For this review, use the dimensioned drawing (mm, ordinates from the lowest corner) and the shaded views. A direction names the side the tool comes from. Give positions to 0.01 mm unless a question says otherwise; leave off trailing zeros. Order: outer loops, then holes, each group sorted by start corner. A loop starts at its lowest first (then second) coordinate and runs counter-clockwise, first axis right, second up. Notation, with made-up numbers: (67, 24.5) - (93, 24.5) arc R26 cw to (93, 61.5) - close; hole circle Ø10 at (82, 62). An arc over 180 degrees is marked (long way). Use a Markdown table: item, result. Add a question column.
1) Clearance check with flat-ended pins moving along their axes: P1, Ø16, axis at y = 9.5, z = 26.5, coming from the +X side; P2, Ø1, axis at y = 16.5, z = 10.5, coming from the -X side; P3, Ø6, axis at x = 12, y = 30.5, coming from the +Z side. State where each tip first meets the part, or that it passes through.
2) We need section C-C on x = 32.5. Write out the cut boundary in (y, z), then the cut area to 3 significant figures.
3) We need section D-D on z = 26.5. Write out the cut boundary in (x, y).
4) We need section B-B on z = 8. Write out the cut boundary in (x, y).
5) Mouldability with a two-part tool opening along X and no side actions: class the marked faces 5, 6, 7 and 8 as released by +X, released by -X, zero draft, split by the parting line, or undercut.
6) Wall thickness on L1, parallel to Z at x = 11, y = 40.25; L2, parallel to Z at x = 14, y = 39.5; L3, parallel to Y at x = 31.5, z = 36.5: over which ranges is each line inside the solid? List them lowest first.
7) Machinability: for the marked faces 1, 2, 3 and 4, which of the approach directions +Z, -Z, +X, -X, +Y, -Y give a long, thin tool a straight path to every point of the face, cutting with its end or side? Answer none if there is none.
8) We need section A-A on z = 3. Write out the cut boundary in (x, y), then the cut area to 3 significant figures.
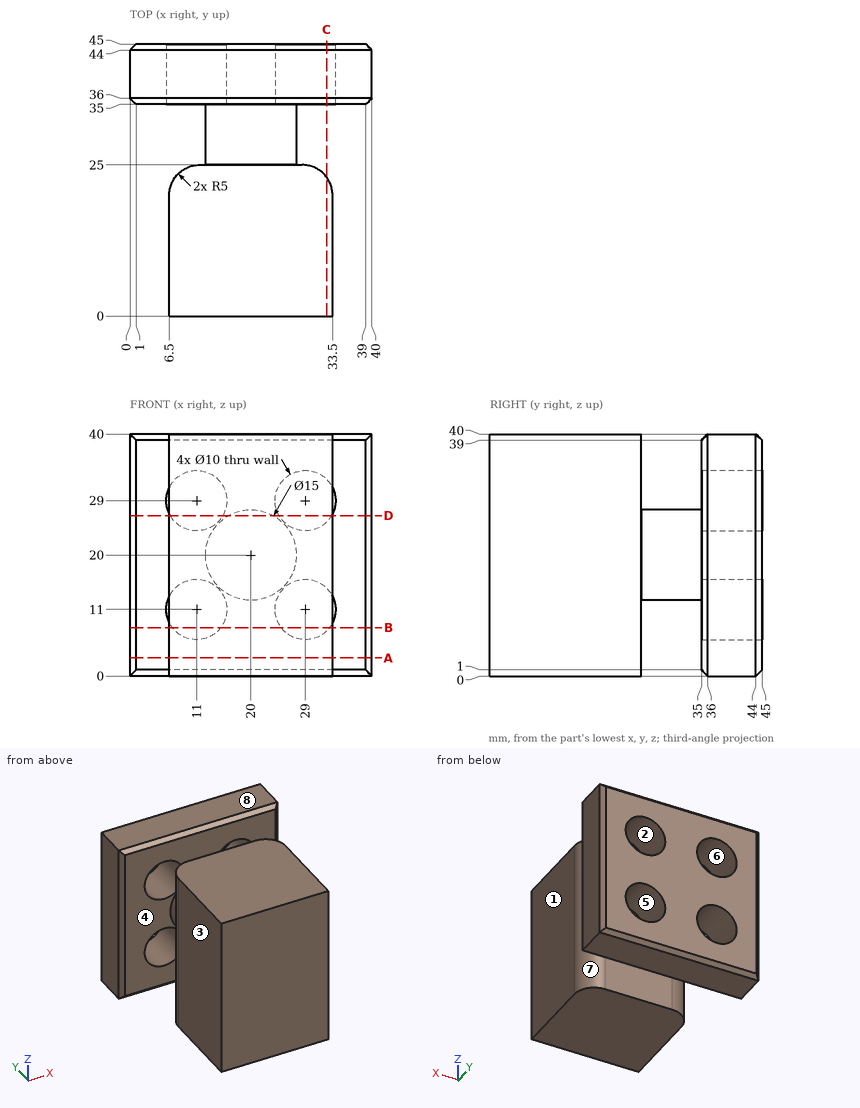
Checked values:
| question | item | result |
|---|---|---|
| 1 | P1 | x = 33.5 |
| 1 | P2 | x = 6.5 |
| 1 | P3 | z = 25.59 |
| 2 | outline | (0, 0) - (23, 0) - (23, 40) - (0, 40) - close; (35, 1) - (36, 0) - (44, 0) - (45, 1) - (45, 7.43) - (35, 7.43) - close; (35, 14.57) - (45, 14.57) - (45, 25.43) - (35, 25.43) - close; (35, 32.57) - (45, 32.57) - (45, 39) - (44, 40) - (36, 40) - (35, 39) - close |
| 2 | area | 1,180 mm² |
| 3 | outline | (0, 36) - (1, 35) - (6.67, 35) - (6.67, 45) - (1, 45) - (0, 44) - close; (6.5, 0) - (33.5, 0) - (33.5, 20) arc R5 ccw to (28.5, 25) - (23.74, 25) - (23.74, 35) - (24.67, 35) - (24.67, 45) - (15.33, 45) - (15.33, 35) - (16.26, 35) - (16.26, 25) - (11.5, 25) arc R5 ccw to (6.5, 20) - close; (33.33, 35) - (39, 35) - (40, 36) - (40, 44) - (39, 45) - (33.33, 45) - close |
| 4 | outline | (0, 36) - (1, 35) - (7, 35) - (7, 45) - (1, 45) - (0, 44) - close; (6.5, 0) - (33.5, 0) - (33.5, 20) arc R5 ccw to (28.5, 25) - (11.5, 25) arc R5 ccw to (6.5, 20) - close; (15, 35) - (25, 35) - (25, 45) - (15, 45) - close; (33, 35) - (39, 35) - (40, 36) - (40, 44) - (39, 45) - (33, 45) - close |
| 5 | face 5 | undercut |
| 5 | face 6 | undercut |
| 5 | face 7 | released by +X |
| 5 | face 8 | zero draft |
| 6 | L1 | 0 to 6, 16 to 24, 34 to 40 |
| 6 | L2 | 0 to 7, 15 to 25, 33 to 40 |
| 6 | L3 | 0 to 24, 35 to 45 |
| 7 | face 1 | +Z, -Z, +X, -Y |
| 7 | face 2 | +Y |
| 7 | face 3 | +Z, -Z, -X, -Y |
| 7 | face 4 | none |
| 8 | outline | (0, 36) - (1, 35) - (39, 35) - (40, 36) - (40, 44) - (39, 45) - (1, 45) - (0, 44) - close; (6.5, 0) - (33.5, 0) - (33.5, 20) arc R5 ccw to (28.5, 25) - (11.5, 25) arc R5 ccw to (6.5, 20) - close |
| 8 | area | 1,060 mm² |
